Design review of the part built by this model. Coordinates are the model's own, in mm. Face numbers are marked on the shaded views. Give positions to 0.01 mm unless a question says otherwise; leave off trailing zeros. Loops run counter-clockwise (first coordinate to the right, second up) from the corner with the lowest first, then second, coordinate; pieces in that order, holes last. Notation, with made-up numbers: (48, -28.75) -> (81, -28.75) arc R28 ccw to (81, 0.25) -> close; hole circle Ø2 at (-37, -8). An arc over 180 degrees is marked (long way). Use a Markdown table: item, result. Add a question column.
1. To check wall thickness, follow line 1 (Y direction, x = 4.5, z = 0); line 2 (X direction, y = -7.25, z = 3.5). State the ranges of each line that lie inside material, in increasing order.
2. Add section D-D (x = 2.5). State the section outline as (y, z) points.
3. Draft analysis for pull direction Z (two halves, no side actions). For the marked faces 1, 2 and 3, state which applies: pulls with the +Z half, pulls with the -Z half, needs draft (parallel to the pull), parting line crosses it, or undercut.
4. Add section C-C (x = 8). State the section outline as (y, z) points, and give its area (3 significant figures).
5. For pin 1 Ø1 at (x, z) = (7, 6.5) entering from +Y; pin 2 Ø2 at (x, y) = (2.5, -1) entering from +Z; pin 3 Ø5 at (x, z) = (12, -6) entering from +Y; pin 4 Ø6 at (y, z) = (0, 0) entering from +X (3 decimals), all flat-tipped, find the tip position at first contact; note any pin that passes through.
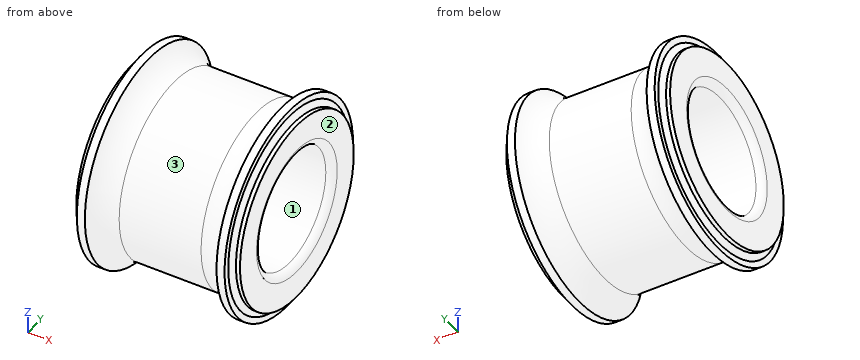
```python
from build123d import *


with BuildPart() as part:
    # Sketch1 → Revolve1 (revolve)
    with BuildSketch(Plane.XY):
        with BuildLine():
            Line((0.6, 5), (13.4, 5))
            ThreePointArc((13.4, 5), (13.824264069, 5.175735931), (14, 5.6))
            Line((14, 5.6), (14, 8.728))
            ThreePointArc((14, 8.728), (13.941421356, 8.869421356), (13.8, 8.928))
            Line((13.8, 8.928), (12.627143625, 8.928))
            ThreePointArc((12.627143625, 8.928), (11.749083664, 7.971770723), (10.5, 7.618))
            Line((10.5, 7.618), (3.5, 7.618))
            ThreePointArc((3.5, 7.618), (2.250916336, 7.971770723), (1.372856375, 8.928))
            Line((1.372856375, 8.928), (0.2, 8.928))
            ThreePointArc((0.2, 8.928), (0.058578644, 8.869421356), (0, 8.728))
            Line((0, 8.728), (0, 5.6))
            ThreePointArc((0, 5.6), (0.175735931, 5.175735931), (0.6, 5))
        make_face()
    revolve(axis=Axis((13.4, 0, 0), (-1, 0, 0)))

    # Sketch2 → Cut-Revolve1 (revolve, cut)
    with BuildSketch(Plane.XY):
        Polygon((0, 7.9), (0.343214094, 7.9), (0.686428188, 8.414), (0.686428188, 8.928), (13.313571812, 8.928), (13.313571812, 8.414), (13.656785906, 7.9), (14, 7.9), (14, 11.828), (0, 11.828), align=None)
    revolve(axis=Axis((14, 0, 0), (-1, 0, 0)), mode=Mode.SUBTRACT)


solid = part.part
```
Taken from the geometry:
| question | item | result |
|---|---|---|
| 1 | line 1 | y = -7.62 to -5, 5 to 7.62 |
| 1 | line 2 | x = 0.44 to 2.13, 11.87 to 13.56 |
| 2 | outline | circle Ø15.68 at (0, 0); hole circle Ø10 at (0, 0) |
| 3 | face 1 | undercut |
| 3 | face 2 | needs draft |
| 3 | face 3 | parting line crosses it |
| 4 | outline | circle Ø15.24 at (0, 0); hole circle Ø10 at (0, 0) |
| 4 | area | 104 mm^2 |
| 5 | pin 1 | stops at y = 4.69 |
| 5 | pin 2 | stops at z = 8.65 |
| 5 | pin 3 | stops at y = 8.18 |
| 5 | pin 4 | passes through |
